from build123d import *

# Parameters (mm, degrees)
SKETCH1_W           = 95.25
SKETCH1_H           = 241.3
BOSS_EXTRUDE1_DEPTH = 6.35
SKETCH2_W           = 6.35
SKETCH2_H           = 12.7
CUT_EXTRUDE1_DEPTH  = 7.35
LPATTERN1_COUNT     = 9
LPATTERN1_PITCH     = 25.4
SKETCH3_R           = 1.75
CUT_EXTRUDE2_DEPTH  = 7.35
SKETCH4_W           = 60.96
SKETCH4_H           = 80.01
CUT_EXTRUDE3_DEPTH  = 7.35
CHAMFER1_SIZE       = 2.54


with BuildPart() as part:
    # Sketch1 → Boss-Extrude1 (new body)
    with BuildSketch(Plane.XY):
        with Locations((47.625, 120.65)):
            Rectangle(SKETCH1_W, SKETCH1_H)
    extrude(amount=BOSS_EXTRUDE1_DEPTH)

    # Sketch2 → Cut-Extrude1 (cut, through all)
    with BuildSketch(Plane.XY.offset(6.35)):
        with Locations((3.175, 222.25)):
            Rectangle(SKETCH2_W, SKETCH2_H)
        with Locations((92.075, 222.25)):
            Rectangle(SKETCH2_W, SKETCH2_H)
    cut_extrude1 = extrude(amount=-CUT_EXTRUDE1_DEPTH, mode=Mode.SUBTRACT)

    # LPattern1: Cut-Extrude1 ×9, 2 skipped
    with Locations(*[(0, -i * LPATTERN1_PITCH, 0) for i in range(1, LPATTERN1_COUNT) if i not in (5, 7)]):
        add(cut_extrude1, mode=Mode.SUBTRACT)

    # Sketch3 → Cut-Extrude2 (cut, through all)
    with BuildSketch(Plane.XY.offset(6.35)):
        with Locations((7.625, 93.85)):
            Circle(SKETCH3_R)
        with Locations((7.625, 45.85)):
            Circle(SKETCH3_R)
        with Locations((87.625, 93.85)):
            Circle(SKETCH3_R)
        with Locations((87.625, 45.85)):
            Circle(SKETCH3_R)
    extrude(amount=-CUT_EXTRUDE2_DEPTH, mode=Mode.SUBTRACT)

    # Sketch4 → Cut-Extrude3 (cut, through all)
    with BuildSketch(Plane.XY.offset(6.35)):
        with Locations((47.625, 74.295)):
            Rectangle(SKETCH4_W, SKETCH4_H)
    extrude(amount=-CUT_EXTRUDE3_DEPTH, mode=Mode.SUBTRACT)

    # Chamfer1
    chamfer1_edges = [part.edges().sort_by_distance(p)[0] for p in [
        (17.145, 114.3, 3.175),
        (78.105, 114.3, 3.175),
        (78.105, 34.29, 3.175),
        (17.145, 34.29, 3.175),
    ]]
    chamfer(chamfer1_edges, length=CHAMFER1_SIZE)


solid = part.part
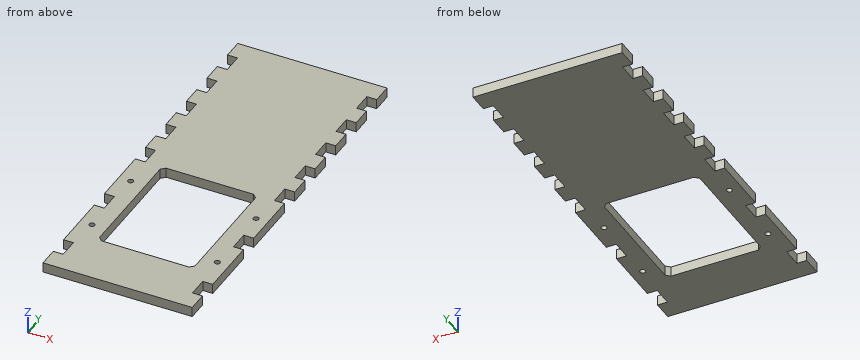
Geometry check sheet. Reference: the model listing, model coordinates, mm. Give positions to 0.01 mm unless a question says otherwise; leave off trailing zeros. Order: outer loops, then holes, each group sorted by start corner. A loop starts at its lowest first (then second) coordinate and runs counter-clockwise, first axis right, second up. Notation, with made-up numbers: (8.5, -25.75) - (65.5, -25.75) arc R13 ccw to (65.5, -20.75) - close; hole circle Ø11 at (-1, 10). An arc over 180 degrees is marked (long way). Answer as a JSON object with one key per item and string values.
(1) Depth check by flat-ended pin: pin 1 Ø1 at (y, z) = (141, 1.5) entering from +X; pin 2 Ø3 at (y, z) = (122, 4.5) entering from -X. Enter the tip coordinate at first touch or a pass-through.
Report:
{"pin 1": "x = 88.9", "pin 2": "x = 6.35"}
(2) Cross-section at B-B (y = 195). Record the cut outline in (x, z).
Report:
{"outline": "(6.35, 0) - (88.9, 0) - (88.9, 6.35) - (6.35, 6.35) - close"}
(3) Cross-section at A-A (x = 41). Record the cut outline in (y, z), then the cut area to 3 significant figures.
Report:
{"outline": "(0, 0) - (34.29, 0) - (34.29, 6.35) - (0, 6.35) - close; (114.3, 0) - (241.3, 0) - (241.3, 6.35) - (114.3, 6.35) - close", "area": "1,020 mm^2"}
(4) Material ranges on line 1 (X direction, y = 93.85, z = 2.5) (3 decimals); line 2 (Y direction, x = 67, z = 3); line 3 (X direction, y = 56, z = 5.25) (3 decimals), recorded low to high.
Report:
{"line 1": "0 to 5.875, 9.375 to 17.145, 78.105 to 85.875, 89.375 to 95.25", "line 2": "0 to 34.29, 114.3 to 241.3", "line 3": "0 to 17.145, 78.105 to 95.25"}
(5) Cross-section at C-C (z = 3.75). State how many separate pieces and enclosed holes the cut face has, then the cut area to 3 significant figures.
Report:
{"separate pieces": "1", "enclosed holes": "5", "area": "17,000 mm^2"}
